from build123d import *

# Parameters (mm, degrees)
F0_R          = 7.9375
F0_R_2        = 4.7625
F1_DEPTH      = 25.4
F1_DEPTH_BACK = 12.7
F3_DEPTH      = 6.858
F4_R          = 11.421726494
F4_R_2        = 5.0513257944
F5_DEPTH      = 7.8232
F5_TAPER      = 25
F6_R          = 14.5288
F6_R_2        = 4.7625
F7_DEPTH      = 3.175
F8_R          = 1.778
F9_DEPTH      = 15.876
F10_R         = 0.325628867
F11_DEPTH     = 25.4
F12_R         = 0.5092148408
F13_DEPTH     = 25.4


with BuildPart() as f1:
    # F0 (on Top) → F1 (new body, two sides)
    with BuildSketch(Plane.XY) as f1_sk:
        Circle(F0_R)
        Circle(F0_R_2, mode=Mode.SUBTRACT)
    extrude(amount=F1_DEPTH)
    extrude(f1_sk.sketch, amount=-F1_DEPTH_BACK)

    # F2 (on face) → F3 (cut)
    with BuildSketch(Plane.XY.offset(25.4)):
        with BuildLine():
            Line((-2.6014847011, 0), (-10.5939569366, 0))
            ThreePointArc((-10.5939569366, 0), (-7.4910587894, -7.4910587894), (0, -10.5939569366))
            Line((0, -10.5939569366), (0, -2.6014847011))
            ThreePointArc((0, -2.6014847011), (-1.8395274733, -1.8395274733), (-2.6014847011, 0))
        make_face()
        with BuildLine():
            ThreePointArc((0, 2.6014847011), (1.8395274733, 1.8395274733), (2.6014847011, 0))
            Line((2.6014847011, 0), (10.5939569366, 0))
            ThreePointArc((10.5939569366, 0), (7.4910587894, 7.4910587894), (0, 10.5939569366))
            Line((0, 10.5939569366), (0, 2.6014847011))
        make_face()
    extrude(amount=-F3_DEPTH, mode=Mode.SUBTRACT)

    # F4 (on face) → F5 (cut)
    with BuildSketch(Plane.XY.offset(25.4)):
        Circle(F4_R)
        Circle(F4_R_2, mode=Mode.SUBTRACT)
    extrude(amount=-F5_DEPTH, taper=F5_TAPER, mode=Mode.SUBTRACT)

    # F6 (on Top) → F7 (join)
    with BuildSketch(Plane.XY):
        Circle(F6_R)
        Circle(F6_R_2, mode=Mode.SUBTRACT)
    extrude(amount=F7_DEPTH)

    # F8 (on face) → F9 (cut, through all)
    with BuildSketch(Plane.XY.offset(3.175)):
        with Locations((0, 11.0998)):
            Circle(F8_R)
        with Locations((9.6127087769, -5.5499)):
            Circle(F8_R)
        with Locations((-9.6127087769, -5.5499)):
            Circle(F8_R)
    extrude(amount=-F9_DEPTH, mode=Mode.SUBTRACT)

    # F10 (on face) → F11 (cut)
    with BuildSketch(Plane.YZ):
        with Locations((5.7785, 20.9641065449)):
            Circle(F10_R)
    extrude(amount=-F11_DEPTH, mode=Mode.SUBTRACT)

    # F12 (on face) → F13 (cut)
    with BuildSketch(Plane(origin=(0, 0, 0), x_dir=(0, -1, 0), z_dir=(-1, 0, 0))):
        with Locations((5.7785, 20.9257006645)):
            Circle(F12_R)
    extrude(amount=-F13_DEPTH, mode=Mode.SUBTRACT)


solid = f1.part
CAD build for the part. Positions are in the model's coordinates, mm. A direction names the side the tool comes from. Coordinates: 2 decimals unless noted, no trailing zeros. Loops run counter-clockwise (first coordinate to the right, second up) from the corner with the lowest first, then second, coordinate; pieces in that order, holes last. Notation, with made-up numbers: (62, -24) - (89, -24) arc R27 ccw to (89, 6) - close; hole circle Ø4 at (62.25, -23). An arc over 180 degrees is marked (long way). Use one line per item in the form item = value. Start each with the question number.
1) Band-saw the part on B-B (z = -1.5). Give the cut face in (x, y) (1 decimal).
2) Tool access for faces 5 (the face through (-6, 0, 21)), 6 (the face through (-1.72, -7.75, 11.31)), 7 (the face through (6, -6, 0)), 8 (the face through (0, 6, 20)): list every direction of +Z, -Z, +X, -X, +Y, -Y with a clear straight run to the whole face (end or side of a thin tool).
3) Band-saw the part on C-C (z = 2.5). Give the cut face in (x, y) (1 decimal), and give its area (3 significant figures).
4) Band-saw the part on A-A (x = -0.75). State how many separate pieces and enclosed holes the cut face has, and give its area (3 significant figures).
5) Flat gauge pins, fed straight in: pin 1 (3.5 mm diameter, centred on x = -7, z = 23.5, fed in from -Y); pin 2 (4.5 mm diameter, centred on x = -9.61, y = -5.55, fed in from -Z); pin 3 (6 mm diameter, centred on y = -7.5, z = -4.5, fed in from +X). Where does each tip first touch, or does it go through?
6) Drill centre lines: L1, parallel to Y at x = 0, z = 0.6; L2, parallel to Y at x = 0, z = 4; L3, parallel to Z at x = -12, y = -1.5 (3 decimals). Where is each one in solid material? Low to high. Write a range as from..to.
7) Two-plate mould, pull along Y, no slides. Class faces 1 (the face through (6, 0, 21)), 2 (the face through (-1.72, -7.75, -6.26)), 3 (the face through (6, -6, 3.175)), 4 (the face through (7.836, -5.472, 1.61)): +Y half, -Y half, draft (parallel to the pull), parting line (faces both ways), or undercut.
Check values:
q1.outline = circle Ø15.9 at (0, 0); hole circle Ø9.5 at (0, 0)
q2.face_5 = +Z, -X, -Y
q2.face_6 = +Z
q2.face_7 = -Z
q2.face_8 = +Z, +X, +Y
q3.outline = circle Ø29.1 at (0, 0); hole circle Ø3.6 at (-9.6, -5.5); hole circle Ø9.5 at (0, 0); hole circle Ø3.6 at (0, 11.1); hole circle Ø3.6 at (9.6, -5.5)
q3.area = 562 mm2
q4.separate_pieces = 3
q4.enclosed_holes = 1
q4.area = 244 mm2
q5.pin_1 = 0
q5.pin_2 = 0
q5.pin_3 = 6.54
q6.L1 = -14.53..-4.76, 4.76..9.32, 12.88..14.53
q6.L2 = -7.94..-4.76, 4.76..7.94
q6.L3 = 0..3.175
q7.face_1 = +Y half
q7.face_2 = parting line
q7.face_3 = draft
q7.face_4 = undercut
